Part model, mm, in its own coordinate system. Face numbers are marked on the shaded views. A direction names the side the tool comes from. Round coordinates to 2 decimals unless told otherwise and drop trailing zeros. Write each loop counter-clockwise with the first axis right and the second up, starting at its lowest first coordinate (ties: lowest second). Pieces come first, ordered by that corner, then holes.
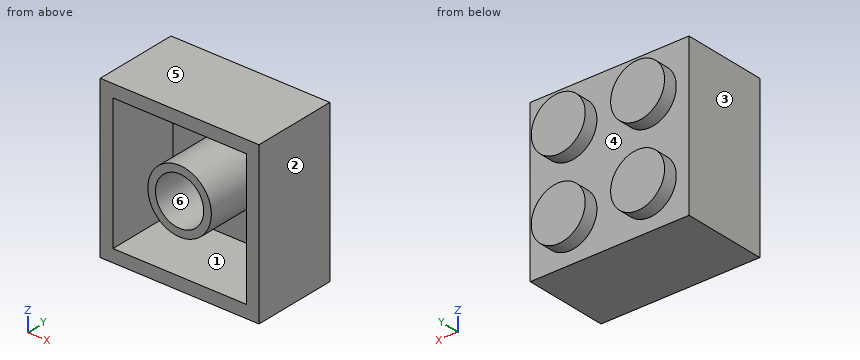
```python
from build123d import *

# Parameters (mm, degrees)
SKETCH1_W           = 15.875
SKETCH1_H           = 15.875
BOSS_EXTRUDE1_DEPTH = 4.2291
SKETCH2_W           = 13.335
SKETCH2_H           = 13.335
SKETCH2_R           = 3.175
SKETCH2_R_2         = 2.413
CUT_EXTRUDE1_DEPTH  = 7.1882
SKETCH3_R           = 2.69875
BOSS_EXTRUDE2_DEPTH = 1.397


with BuildPart() as part:
    # Sketch1 → Boss-Extrude1 (new body, symmetric)
    with BuildSketch(Plane(origin=(0, 0, 0), x_dir=(1, 0, 0), z_dir=(0, 1, 0))):
        Rectangle(SKETCH1_W, SKETCH1_H)
    extrude(amount=BOSS_EXTRUDE1_DEPTH, both=True)

    # Sketch2 → Cut-Extrude1 (cut)
    with BuildSketch(Plane.XZ.offset(4.2291)):
        Rectangle(SKETCH2_W, SKETCH2_H)
        Circle(SKETCH2_R, mode=Mode.SUBTRACT)
        Circle(SKETCH2_R_2)
    extrude(amount=-CUT_EXTRUDE1_DEPTH, mode=Mode.SUBTRACT)

    # Sketch3 → Boss-Extrude2 (add)
    with BuildSketch(Plane(origin=(0, 4.2291, 0), x_dir=(1, 0, 0), z_dir=(0, 1, 0))):
        with Locations((3.96875, -3.96875)):
            Circle(SKETCH3_R)
        with Locations((3.96875, 3.96875)):
            Circle(SKETCH3_R)
        with Locations((-3.96875, -3.96875)):
            Circle(SKETCH3_R)
        with Locations((-3.96875, 3.96875)):
            Circle(SKETCH3_R)
    extrude(amount=BOSS_EXTRUDE2_DEPTH)


solid = part.part
```
Q1. Cut at C-C on z = 0. Write the cut outline in (x, y) (1 decimal), plus the area to 3 significant figures.
Values follow:
outline: (-7.9, -4.2) - (-6.7, -4.2) - (-6.7, 3) - (-3.2, 3) - (-3.2, -4.2) - (-2.4, -4.2) - (-2.4, 3) - (2.4, 3) - (2.4, -4.2) - (3.2, -4.2) - (3.2, 3) - (6.7, 3) - (6.7, -4.2) - (7.9, -4.2) - (7.9, 4.2) - (-7.9, 4.2) - close
area: 49.4 mm2
Q2. Which spindle directions (+Z, -Z, +X, -X, +Y, -Y) get a long thin tool onto all of the face, cutting with end or side? Do the marked faces 4, 5 and 6. Say none if no direction does.
Values follow:
face 4: +Y
face 5: +Z, +X, -X, +Y, -Y
face 6: -Y
Q3. Wall check: L1, parallel to Z at x = 0, y = 0.5 (1 decimal); L2, parallel to X at y = -3, z = -5.5. Give the ranges that are in metal, low to high.
Values follow:
L1: z = -7.9 to -6.7, -3.2 to -2.4, 2.4 to 3.2, 6.7 to 7.9
L2: x = -7.94 to -6.67, 6.67 to 7.94
Q4. Drop a flat-ended pin along its axis: pin 1 (4 mm diameter, centred on x = 0, z = 0, fed in from -Y). Give the stop position or say it passes through.
Values follow:
pin 1: stops at y = 2.96
Q5. Cut at D-D on x = -2.75. Write the cut outline in (y, z).
Values follow:
outline: (-4.23, -7.94) - (4.23, -7.94) - (4.23, -6.38) - (5.63, -6.38) - (5.63, -1.56) - (4.23, -1.56) - (4.23, 1.56) - (5.63, 1.56) - (5.63, 6.38) - (4.23, 6.38) - (4.23, 7.94) - (-4.23, 7.94) - (-4.23, 6.67) - (2.96, 6.67) - (2.96, 1.59) - (-4.23, 1.59) - (-4.23, -1.59) - (2.96, -1.59) - (2.96, -6.67) - (-4.23, -6.67) - close
Q6. Cut at B-B on x = 0. Write the cut outline in (y, z) (1 decimal).
Values follow:
outline: (-4.2, -7.9) - (4.2, -7.9) - (4.2, 7.9) - (-4.2, 7.9) - (-4.2, 6.7) - (3, 6.7) - (3, 3.2) - (-4.2, 3.2) - (-4.2, 2.4) - (3, 2.4) - (3, -2.4) - (-4.2, -2.4) - (-4.2, -3.2) - (3, -3.2) - (3, -6.7) - (-4.2, -6.7) - close
Q7. Cut at A-A on y = -1. State how many separate pieces and enclosed holes the cut face has, plus the area to 3 significant figures.
Values follow:
separate pieces: 2
enclosed holes: 2
area: 87.6 mm2
Q8. Mould opens along X. For the marked faces 1, 2 and 3 say: +X half, -X half, draft (parallel to the pull), parting line (faces both ways), or undercut.
Values follow:
face 1: undercut
face 2: +X half
face 3: -X half
